Work out the finished part from the listing and answer in its coordinate system (mm). A direction names the side the tool comes from. Give positions to 0.01 mm unless a question says otherwise; leave off trailing zeros. Write each loop counter-clockwise with the first axis right and the second up, starting at its lowest first coordinate (ties: lowest second). Pieces come first, ordered by that corner, then holes. Notation, with made-up numbers: (45, -31) - (77, -31) arc R28 ccw to (77, 8) - close; hole circle Ø11 at (86, 68). An arc over 180 degrees is marked (long way). Write item = value, one per line.
from build123d import *

# Parameters (mm, degrees)
SKETCH2_W           = 15.88
SKETCH2_H           = 21.21
BOSS_EXTRUDE1_DEPTH = 13.89
SKETCH3_R           = 5.145
BOSS_EXTRUDE2_DEPTH = 9.53
SKETCH4_R           = 3.17
BOSS_EXTRUDE3_DEPTH = 13
CUT_EXTRUDE1_DEPTH  = 10


with BuildPart() as part:
    # Sketch2 → Boss-Extrude1 (new body)
    with BuildSketch(Plane.XY):
        with Locations((7.94, 10.605)):
            Rectangle(SKETCH2_W, SKETCH2_H)
    extrude(amount=BOSS_EXTRUDE1_DEPTH)

    # Sketch3 → Boss-Extrude2 (add)
    with BuildSketch(Plane.XY.offset(13.89)):
        with Locations((7.94, 12)):
            Circle(SKETCH3_R)
    extrude(amount=BOSS_EXTRUDE2_DEPTH)

    # Sketch4 → Boss-Extrude3 (add)
    with BuildSketch(Plane.XY.offset(23.42)):
        with Locations(Location((7.94, 12, 0), (0, 0, 180))):
            Circle(SKETCH4_R)
    extrude(amount=BOSS_EXTRUDE3_DEPTH)

    # Sketch5 → Cut-Extrude1 (cut)
    with BuildSketch(Plane.XY.offset(36.42)):
        with BuildLine():
            Line((10.099, 14.327948453), (10.099, 9.672051547))
            ThreePointArc((10.099, 9.672051547), (11.115, 12), (10.099, 14.327948453))
        make_face()
    extrude(amount=-CUT_EXTRUDE1_DEPTH, mode=Mode.SUBTRACT)


solid = part.part
1. Find section D-D, the plane x = 6. Give the vertices of the cut face in (y, z).
Solution:
outline = (0, 0) - (21.21, 0) - (21.21, 13.89) - (16.77, 13.89) - (16.77, 23.42) - (14.51, 23.42) - (14.51, 36.42) - (9.49, 36.42) - (9.49, 23.42) - (7.23, 23.42) - (7.23, 13.89) - (0, 13.89) - close
2. Given pin 1 (1.4 mm diameter, centred on y = 11, z = 32.5, fed in from +X); pin 2 (5 mm diameter, centred on x = 14, y = 14.5, fed in from +Z); pin 3 (1.5 mm diameter, centred on y = 9.5, z = 19, fed in from +X), each flat-ended and moving along its own axis, determine where each tip first touches the part or whether it passes through.
Solution:
pin_1 = 10.1
pin_2 = 23.42
pin_3 = 12.78
3. A tool of negligible diameter and unlimited length cuts with its end or side. For faces 1 (the cylindrical face through (5.01, 13.21, 29.83)), 2 (the flat face through (10.099, 12, 31)), 3 (the flat face through (0, 10, 7)), from which of +Z, -Z, +X, -X, +Y, -Y can it reach the whole face along a straight path? Write none if from no direction.
Solution:
face_1 = +Z
face_2 = +Z, +X, +Y, -Y
face_3 = +Z, -Z, -X, +Y, -Y
4. Find section C-C, the plane z = 20.5. Give the vertices of the cut face in (x, y) (3 decimals).
Solution:
outline = circle Ø10.29 at (7.94, 12)
5. Find section B-B, the plane y = 12. Give the vertices of the cut face in (x, z) (3 decimals).
Solution:
outline = (0, 0) - (15.88, 0) - (15.88, 13.89) - (13.085, 13.89) - (13.085, 23.42) - (11.11, 23.42) - (11.11, 26.42) - (10.099, 26.42) - (10.099, 36.42) - (4.77, 36.42) - (4.77, 23.42) - (2.795, 23.42) - (2.795, 13.89) - (0, 13.89) - close
6. Find section A-A, the plane x = 7.94. Give the vertices of the cut face in (y, z) (3 decimals), then the cut area to 3 significant figures.
Solution:
outline = (0, 0) - (21.21, 0) - (21.21, 13.89) - (17.145, 13.89) - (17.145, 23.42) - (15.17, 23.42) - (15.17, 36.42) - (8.83, 36.42) - (8.83, 23.42) - (6.855, 23.42) - (6.855, 13.89) - (0, 13.89) - close
area = 475 mm^2
7. Straight lines are drawn through the part: line 1 (Z direction, x = 1.75, y = 20); line 2 (Z direction, x = 10.75, y = 8.75); line 3 (X direction, y = 8, z = 14). For each, find the intervals that lie inside material, in ascending order.
Solution:
line_1 = 0 to 13.89
line_2 = 0 to 23.42
line_3 = 4.7 to 11.18
